Autodesk Inventor part; units mm, degrees
ref_plane "YZ Plane" through (0, 0, 0) normal (1, 0, 0) x (0, 1, 0)
ref_plane "XZ Plane" through (0, 0, 0) normal (0, 1, 0) x (-1, 0, 0)
ref_plane "XY Plane" through (0, 0, 0) normal (0, 0, 1) x (1, 0, 0)
sketch "Sketch1" plane through (0, 0, 0) normal (0, 0, 1) x (1, 0, 0)
  line L0 (-50, -39.5) -> (50, -39.5)
  line L1 (50, -39.5) -> (50, 39.5)
  line L2 (50, 39.5) -> (-50, 39.5)
  line L3 (-50, 39.5) -> (-50, -39.5)
  line L4 (-50, -39.5) -> (50, 39.5) construction
  line L5 (50, -39.5) -> (-50, 39.5) construction
  point P0 (0, 0)
  dimension "d0" = 100
  dimension "d1" = 79
extrude "Extrusion1" add sketch "Sketch1" along normal blind 2
sketch "Sketch3" plane through (0, 0, 2) normal (0, 0, 1) x (1, 0, 0)
  circle A0 centre (-40, 36) radius 1.25
  circle A1 centre (46.5, 36) radius 1.25
  circle A2 centre (46.5, -22.7) radius 1.25
  line L0 (-50, 39.5) -> (-50, -39.5)
  line L1 (50, 39.5) -> (-50, 39.5)
  line L2 (50, -39.5) -> (50, 39.5)
  line L3 (-50, -39.5) -> (50, -39.5)
  point P0 (0, 0)
  dimension "d6" = 2.5
  dimension "d7" = 2.5
  dimension "d8" = 2.5
  dimension "d9" = 10
  dimension "d10" = 3.5
  dimension "d11" = 3.5
  dimension "d12" = 3.5
  dimension "d13" = 3.5
  dimension "d14" = 16.8
extrude "Extrusion2" cut sketch "Sketch3" against normal blind 2 contours A0 | A1 | A2
fillet "Fillet1" radius 2 3 edges at (50, -39.5, 1) (50, 39.5, 1) (-50, 39.5, 1)
sketch "Sketch4" plane through (0, 0, 2) normal (0, 0, 1) x (1, 0, 0)
  arc A0 (-48, 39.5) -> (-50, 37.5) centre (-48, 37.5) ccw
  line L0 (-50, 37.5) -> (-50, -39.5)
  line L1 (-50, -39.5) -> (48, -39.5)
  arc A1 (48, -39.5) -> (50, -37.5) centre (48, -37.5) ccw
  line L2 (50, -37.5) -> (50, 37.5)
  arc A2 (50, 37.5) -> (48, 39.5) centre (48, 37.5) ccw
  line L3 (48, 39.5) -> (-48, 39.5)
  circle A3 centre (-40, 36) radius 1.25
  circle A4 centre (46.5, 36) radius 1.25
  circle A5 centre (46.5, -22.7) radius 1.25
  line L4 (-50, -39.5) -> (48, -39.5)
  line L5 (48, 39.5) -> (-48, 39.5)
  line L6 (-40, -39.5) -> (40, -39.5)
  line L7 (40, -39.5) -> (40, 39.5)
  line L8 (40, 39.5) -> (-40, 39.5)
  line L9 (-40, 39.5) -> (-40, -39.5)
  point P0 (0, 0)
  dimension "d18" = 10
  dimension "d19" = 10
equation "\"d7\" = d6"
equation "\"d8\" = d6"
equation "\"d11\" = d10"
equation "\"d12\" = d11"
equation "\"d13\" = d12"
equation "\"d19\" = d18"
properties part number "NanoHolder"
Read the model definition and answer for the solid it produces. Units are mm, in the model's axes. Coordinates: 2 decimals unless noted, no trailing zeros. Order: outer loops, then holes, each group sorted by start corner. A loop starts at its lowest first (then second) coordinate and runs counter-clockwise, first axis right, second up. Notation, with made-up numbers: (76.25, 15) - (103.25, 15) arc R11 ccw to (103.25, 26) - close; hole circle Ø2 at (71.25, 24.5). An arc over 180 degrees is marked (long way). Use one line per item in the form item = value.
(1) For a pull along X with two mould halves and no side action, classify faces 1 (the face through (50, -1, 1)), 2 (the face through (-50, 0, 1)), 3 (the face through (-2, -39.5, 1)), 4 (the face through (46.23, -23.92, 1.01)) as pulls with the +X half, pulls with the -X half, needs draft (parallel to the pull), parting line crosses it, or undercut.
Computed values:
face_1 = pulls with the +X half
face_2 = pulls with the -X half
face_3 = needs draft
face_4 = undercut
(2) Section B-B, the plane x = -40 is taken. Give the vertices of the cut face in (y, z).
Computed values:
outline = (-39.5, 0) - (34.75, 0) - (34.75, 2) - (-39.5, 2) - close; (37.25, 0) - (39.5, 0) - (39.5, 2) - (37.25, 2) - close
(3) Straight lines are drawn through the part: L1, parallel to Y at x = 46.5, z = 0.8; L2, parallel to Y at x = -40, z = 1.1; L3, parallel to Y at x = -40.5, z = 0.85. For each, find the intervals that lie inside material, in ascending order.
Computed values:
L1 = -39.5 to -23.95, -21.45 to 34.75, 37.25 to 39.5
L2 = -39.5 to 34.75, 37.25 to 39.5
L3 = -39.5 to 34.85, 37.15 to 39.5
(4) Section A-A, the plane y = -22.7 is taken. Give the vertices of the cut face in (x, z), then the cut area to 3 significant figures.
Computed values:
outline = (-50, 0) - (45.25, 0) - (45.25, 2) - (-50, 2) - close; (47.75, 0) - (50, 0) - (50, 2) - (47.75, 2) - close
area = 195 mm²
(5) Section C-C, the plane y = 36 is taken. Give the vertices of the cut face in (x, z), then the cut area to 3 significant figures.
Computed values:
outline = (-50, 0) - (-41.25, 0) - (-41.25, 2) - (-50, 2) - close; (-38.75, 0) - (45.25, 0) - (45.25, 2) - (-38.75, 2) - close; (47.75, 0) - (50, 0) - (50, 2) - (47.75, 2) - close
area = 190 mm²
(6) Section D-D, the plane x = 46.5 is taken. Give the vertices of the cut face in (y, z).
Computed values:
outline = (-39.5, 0) - (-23.95, 0) - (-23.95, 2) - (-39.5, 2) - close; (-21.45, 0) - (34.75, 0) - (34.75, 2) - (-21.45, 2) - close; (37.25, 0) - (39.5, 0) - (39.5, 2) - (37.25, 2) - close
